```python
from build123d import *

# Parameters (mm, degrees)
SKETCH1_R                = 20
BOSS_EXTRUDE1_DEPTH      = 500
BOSS_EXTRUDE2_DEPTH      = 15
BOSS_EXTRUDE3_DEPTH      = 35
BOSS_EXTRUDE3_DEPTH_BACK = 35
SKETCH3_R                = 10


with BuildPart() as part:
    # Sketch1 → Boss-Extrude1 (new body)
    with BuildSketch(Plane.XY):
        Circle(SKETCH1_R)
    extrude(amount=BOSS_EXTRUDE1_DEPTH)

    # Sketch2 → Boss-Extrude2 (add, symmetric)
    with BuildSketch(Plane(origin=(0, 0, 0), x_dir=(1, 0, 0), z_dir=(0, 1, 0))):
        Polygon((-25, 0), (25, 0), (25, 40), (15, 65), (-15, 65), (-25, 40), align=None)
    extrude(amount=BOSS_EXTRUDE2_DEPTH, both=True)

    # Sketch3 → Boss-Extrude3 (add, two sides: drawn at the far end of the back side and taken through both)
    with BuildSketch(Plane(origin=(0, 0, 0), x_dir=(1, 0, 0), z_dir=(0, 1, 0)).offset(-BOSS_EXTRUDE3_DEPTH_BACK)):
        with Locations(Location((0, 40, 0), (0, 0, 270))):
            Circle(SKETCH3_R)
    extrude(amount=BOSS_EXTRUDE3_DEPTH + BOSS_EXTRUDE3_DEPTH_BACK)


solid = part.part
```
Model file for the job. Use its own axes, mm. A direction names the side the tool comes from. Round coordinates to 2 decimals unless told otherwise and drop trailing zeros. Loops run counter-clockwise (first coordinate to the right, second up) from the corner with the lowest first, then second, coordinate; pieces in that order, holes last. Notation, with made-up numbers: M -6.5,5.5 L 24.5,5.5 A4 ccw 24.5,12.5 Z; hole C 22,56 d6. An arc over 180 degrees is marked long. Put each result on its own line as item: value. Start each with the question number.
Item 1: Cut at D-D (y = -5.5). List the corners of the cut face in (x, z), then the cut area to 3 significant figures.
Item 2: Drill centre lines: line 1 along Y through (x, z) = (0.5, 101.5); line 2 along X through (y, z) = (-2, 347.5). Where is each one in solid material? Low to high.
Item 3: Cut at C-C (z = -19.5). List the corners of the cut face in (x, y), then the cut area to 3 significant figures.
Item 4: Cut at B-B (y = -26.5). List the corners of the cut face in (x, z), then the cut area to 3 significant figures.
Item 5: 3-axis set-ups, long thin cutter, end or side, ignore diameter. For faces 1 (the face through (0, -25, -50)), 2 (the face through (22, 0, 0)), 3 (the face through (-4.336, -19.524, 246.5)), 4 (the face through (0, 25, -50)): which of +Z, -Z, +X, -X, +Y, -Y reach the whole face in a straight line?
Item 6: Mould opens along Z. For faces 5 (the face through (-19.93, 0.21, -52.68)), 6 (the face through (0, -15, -26)), 7 (the face through (0, 15, -26)), 8 (the face through (-22, 0, 0)) say: released by +Z, released by -Z, zero draft, split by the parting line, or undercut.
Item 7: Cut at A-A (x = 5). List the corners of the cut face in (y, z).
Item 8: Drop flat-ended pins along their axis: P1, Ø1, axis at y = 7, z = 305, coming from the -X side; P2, Ø10, axis at x = 2, z = 438.5, coming from the -Y side; P3, Ø2, axis at y = -8, z = 127, coming from the +X side (3 decimals). Give the stop position or say it passes through.
Answer block:
1. outline: M -25,-40 L -15,-65 L 15,-65 L 25,-40 L 25,0 L 19.23,0 L 19.23,500 L -19.23,500 L -19.23,0 L -25,0 Z
1. area: 22,200 mm2
2. line 1: -19.99 to 19.99
2. line 2: -19.9 to 19.9
3. outline: M -25,-15 L 25,-15 L 25,15 L -25,15 Z
3. area: 1,500 mm2
4. outline: C 0,-40 d20
4. area: 314 mm2
5. face 1: -Y
5. face 2: +Z, +X
5. face 3: +Z
5. face 4: +Y
6. face 5: released by -Z
6. face 6: undercut
6. face 7: undercut
6. face 8: released by +Z
7. outline: M -35,-48.66 L -15,-48.66 L -15,-65 L 15,-65 L 15,-48.66 L 35,-48.66 L 35,-31.34 L 15,-31.34 L 15,0 L 19.36,0 L 19.36,500 L -19.36,500 L -19.36,0 L -15,0 L -15,-31.34 L -35,-31.34 Z
8. P1: x = -18.91
8. P2: y = -20
8. P3: x = 18.735
